from build123d import *

# Parameters (mm, degrees)
SKETCH2_R           = 2
BOSS_EXTRUDE1_DEPTH = 3
SKETCH3_W           = 5
SKETCH3_H           = 15
CUT_EXTRUDE1_DEPTH  = 3


with BuildPart() as part:
    # Sketch2 → Boss-Extrude1 (new body)
    with BuildSketch(Plane.XY):
        with BuildLine():
            Line((0, 94), (0, 59.5))
            Line((0, 59.5), (162, 59.5))
            Line((162, 59.5), (162, 114))
            Line((162, 114), (83, 114))
            ThreePointArc((83, 114), (81, 112), (79, 114))
            Line((79, 114), (25, 114))
            Line((25, 114), (25, 104))
            Line((25, 104), (15, 94))
            Line((15, 94), (0, 94))
        make_face()
        with BuildLine():
            Line((83, 114), (162, 114))
            Line((162, 114), (162, 119))
            Line((162, 119), (25, 119))
            Line((25, 119), (25, 114))
            Line((25, 114), (79, 114))
            ThreePointArc((79, 114), (81, 116), (83, 114))
        make_face()
        with BuildLine():
            Line((162, 119), (162, 114))
            Line((162, 114), (241, 114))
            ThreePointArc((241, 114), (243, 116), (245, 114))
            Line((245, 114), (299, 114))
            Line((299, 114), (299, 119))
            Line((299, 119), (162, 119))
        make_face()
        with BuildLine():
            Line((162, 114), (162, 59.5))
            Line((162, 59.5), (324, 59.5))
            Line((324, 59.5), (324, 94))
            Line((324, 94), (309, 94))
            Line((309, 94), (299, 104))
            Line((299, 104), (299, 114))
            Line((299, 114), (245, 114))
            ThreePointArc((245, 114), (243, 112), (241, 114))
            Line((241, 114), (162, 114))
        make_face()
        Polygon((162, 59.5), (162, 0), (299, 0), (299, 15), (309, 25), (324, 25), (324, 59.5), align=None)
        with Locations((243, 5)):
            Circle(SKETCH2_R, mode=Mode.SUBTRACT)
        Polygon((25, 15), (25, 0), (162, 0), (162, 59.5), (0, 59.5), (0, 25), (15, 25), align=None)
        with Locations((81, 5)):
            Circle(SKETCH2_R, mode=Mode.SUBTRACT)
    extrude(amount=BOSS_EXTRUDE1_DEPTH)

    # Sketch3 → Cut-Extrude1 (cut)
    with BuildSketch(Plane.XY.offset(3)):
        with Locations((159.5, 7.5)):
            Rectangle(SKETCH3_W, SKETCH3_H)
        with Locations((164.5, 7.5)):
            Rectangle(SKETCH3_W, SKETCH3_H)
    extrude(amount=-CUT_EXTRUDE1_DEPTH, mode=Mode.SUBTRACT)


solid = part.part
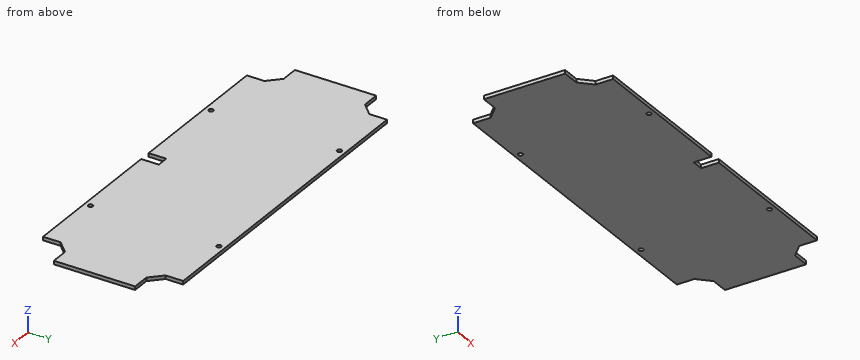
Source: CAD feature listing. Evaluate the final solid. Frame: model axes, mm. Give positions to 0.01 mm unless a question says otherwise; leave off trailing zeros. Loops run counter-clockwise (first coordinate to the right, second up) from the corner with the lowest first, then second, coordinate; pieces in that order, holes last. Notation, with made-up numbers: (52.25, -20.5) -> (70.25, -20.5) arc R14 cw to (70.25, -1.5) -> close; hole circle Ø9 at (13, 69.5). An arc over 180 degrees is marked (long way). Use a Markdown table: item, result. Add a question column.
1) Section query B-B, the plane y = 108. Return the cut outline in (x, z).
2) Section query C-C, the plane y = 20. Return the cut outline in (x, z), then the cut area to 3 significant figures.
3) First-contact query: pin 1 (1.5 mm diameter, centred on y = 5, z = 1, fed in from -X); pin 2 (1.5 mm diameter, centred on x = 10.5, z = 2, fed in from +Y); pin 3 (0.9 mm diameter, centred on y = 7, z = 2, fed in from +X). Flat tips, straight axial feed; report the tip coordinate or a pass-through.
4) Line query: line 1 along Y through (x, z) = (243, 1.5); line 2 along X through (y, z) = (12, 1.85); line 3 along X through (y, z) = (113, 1.65). Output: solid intervals per line, ascending. Write a range as [from, to].
5) Section query A-A, the plane z = 1.85. Return the cut outline in (x, y).
Numbers:
| question | item | result |
|---|---|---|
| 1 | outline | (25, 0) -> (299, 0) -> (299, 3) -> (25, 3) -> close |
| 2 | outline | (20, 0) -> (304, 0) -> (304, 3) -> (20, 3) -> close |
| 2 | area | 852 mm2 |
| 3 | pin 1 | stops at x = 25 |
| 3 | pin 2 | stops at y = 94 |
| 3 | pin 3 | stops at x = 299 |
| 4 | line 1 | y = [0, 3], [7, 112], [116, 119] |
| 4 | line 2 | x = [25, 157], [167, 299] |
| 4 | line 3 | x = [25, 79.27], [82.73, 241.27], [244.73, 299] |
| 5 | outline | (0, 25) -> (15, 25) -> (25, 15) -> (25, 0) -> (157, 0) -> (157, 15) -> (167, 15) -> (167, 0) -> (299, 0) -> (299, 15) -> (309, 25) -> (324, 25) -> (324, 94) -> (309, 94) -> (299, 104) -> (299, 119) -> (25, 119) -> (25, 104) -> (15, 94) -> (0, 94) -> close; hole circle Ø4 at (81, 5); hole circle Ø4 at (81, 114); hole circle Ø4 at (243, 5); hole circle Ø4 at (243, 114) |
